from build123d import *

# Parameters (mm, degrees)
SKETCH1_W                = 50
SKETCH1_H                = 60
BOSS_EXTRUDE1_DEPTH      = 25
CUT_EXTRUDE1_START       = -16.25
SKETCH2_R                = 21
CUT_EXTRUDE1_DEPTH       = 17.5
CUT_EXTRUDE2_START       = -12
SKETCH3_R                = 7.5
CUT_EXTRUDE2_DEPTH       = 26
SKETCH4_R                = 5
CUT_EXTRUDE3_DEPTH       = 4
SKETCH10_W               = 11
SKETCH10_H               = 10
CUT_EXTRUDE9_DEPTH       = 11
SKETCH11_R               = 2.25
CUT_EXTRUDE10_DEPTH      = 50.398886627
SKETCH12_R               = 2
CUT_EXTRUDE11_DEPTH      = 50.371044145
SKETCH13_R               = 3.5
CUT_EXTRUDE12_DEPTH      = 50.371044145
CHAMFER1_SIZE            = 3
FILLET1_R                = 4
SKETCH14_R               = 1.8
CUT_EXTRUDE13_DEPTH      = 10
CUT_EXTRUDE14_DEPTH      = 7
BOSS_EXTRUDE2_DEPTH      = 5
CHAMFER2_SIZE            = 3
FILLET2_R                = 1
CUT_EXTRUDE15_DEPTH      = 66.030761952
CUT_EXTRUDE15_DEPTH_BACK = 66.030761952
SKETCH17_R               = 6
SKETCH21_R               = 7.75
CUT_EXTRUDE16_DEPTH      = 8
SKETCH22_W               = 20
SKETCH22_H               = 10
BOSS_EXTRUDE3_DEPTH      = 5
SKETCH23_R               = 3.25
CUT_EXTRUDE17_DEPTH      = 5
SKETCH24_R               = 5
CUT_EXTRUDE18_DEPTH      = 4
FILLET4_R                = 5
SKETCH25_R               = 1.5
CUT_EXTRUDE19_DEPTH      = 8
SKETCH26_R               = 3.6
CUT_EXTRUDE20_DEPTH      = 10


with BuildPart() as part:
    # Sketch1 → Boss-Extrude1 (new body)
    with BuildSketch(Plane(origin=(0, 0, 0), x_dir=(1, 0, 0), z_dir=(0, 1, 0))):
        Rectangle(SKETCH1_W, SKETCH1_H)
    extrude(amount=BOSS_EXTRUDE1_DEPTH)

    # Sketch2 → Cut-Extrude1 (cut)
    with BuildSketch(Plane.ZY.offset(25).offset(CUT_EXTRUDE1_START)):
        with Locations((0, 25)):
            Circle(SKETCH2_R)
    extrude(amount=-CUT_EXTRUDE1_DEPTH, mode=Mode.SUBTRACT)

    # Sketch3 → Cut-Extrude2 (cut)
    with BuildSketch(Plane.ZY.offset(25).offset(CUT_EXTRUDE2_START)):
        with Locations((0, 25)):
            Circle(SKETCH3_R)
    extrude(amount=-CUT_EXTRUDE2_DEPTH, mode=Mode.SUBTRACT)

    # Sketch4 → Cut-Extrude3 (cut)
    with BuildSketch(Plane.XY.offset(30)):
        with Locations((0, 25)):
            Circle(SKETCH4_R)
    extrude(amount=-CUT_EXTRUDE3_DEPTH, mode=Mode.SUBTRACT)

    # Sketch10 → Cut-Extrude9 (cut)
    with BuildSketch(Plane(origin=(25, 0, 0), x_dir=(0, 0, -1), z_dir=(1, 0, 0))):
        with Locations((-10, 5)):
            Rectangle(SKETCH10_W, SKETCH10_H)
        with Locations((10, 5)):
            Rectangle(SKETCH10_W, SKETCH10_H)
    cut_extrude9 = extrude(amount=-CUT_EXTRUDE9_DEPTH, mode=Mode.SUBTRACT)

    # Sketch11 → Cut-Extrude10 (cut, symmetric)
    with BuildSketch(Plane(origin=(0, 0, -4.5), x_dir=(-1, 0, 0), z_dir=(0, 0, -1))):
        with Locations(Location((-21, 5, 0), (0, 0, 90))):
            Circle(SKETCH11_R)
    cut_extrude10 = extrude(amount=CUT_EXTRUDE10_DEPTH, both=True, mode=Mode.SUBTRACT)

    # Mirror1: Cut-Extrude9, Cut-Extrude10 across plane
    add(cut_extrude9.mirror(Plane(origin=(0, 0, 0), x_dir=(0, 0, 1), z_dir=(1, 0, 0))), mode=Mode.SUBTRACT)
    add(cut_extrude10.mirror(Plane(origin=(0, 0, 0), x_dir=(0, 0, 1), z_dir=(1, 0, 0))), mode=Mode.SUBTRACT)

    # Sketch12 → Cut-Extrude11 (cut, symmetric)
    with BuildSketch(Plane(origin=(0, -2.5, 2.5), x_dir=(1, 0, 0), z_dir=(0, -0.7071067811865475, 0.7071067811865477))):
        with Locations(Location((20, 33.890872965, 0), (0, 0, 270))):
            Circle(SKETCH12_R)
        with Locations(Location((-20, 33.890872965, 0), (0, 0, 270))):
            Circle(SKETCH12_R)
    cut_extrude11 = extrude(amount=CUT_EXTRUDE11_DEPTH, both=True, mode=Mode.SUBTRACT)

    # Sketch13 → Cut-Extrude12 (cut, through all)
    with BuildSketch(Plane(origin=(0, -2.5, 2.5), x_dir=(1, 0, 0), z_dir=(0, -0.7071067811865475, 0.7071067811865477))):
        with Locations(Location((-20, 33.890872965, 0), (0, 0, 90))):
            Circle(SKETCH13_R)
        with Locations(Location((20, 33.890872965, 0), (0, 0, 90))):
            Circle(SKETCH13_R)
    cut_extrude12 = extrude(amount=CUT_EXTRUDE12_DEPTH, mode=Mode.SUBTRACT)

    # Mirror3: Cut-Extrude11, Cut-Extrude12 across plane
    add(cut_extrude11.mirror(Plane.XY), mode=Mode.SUBTRACT)
    add(cut_extrude12.mirror(Plane.XY), mode=Mode.SUBTRACT)

    # Chamfer1
    # the kernel refuses this chamfer: 3 mm, written as the material it takes off along each edge
    with BuildSketch(Plane(origin=(25, -7.715048964, -30), x_dir=(-1, 0, 0), z_dir=(0, 1, 0))) as chamfer1_piece_1:
        Polygon((CHAMFER1_SIZE, 0), (0, CHAMFER1_SIZE), (0, 0), align=None)
    extrude(amount=40.430097928, mode=Mode.SUBTRACT)
    with BuildSketch(Plane(origin=(-25, -7.715048964, -30), x_dir=(1, 0, 0), z_dir=(0, 1, 0))) as chamfer1_piece_2:
        Polygon((CHAMFER1_SIZE, 0), (0, -CHAMFER1_SIZE), (0, 0), align=None)
    extrude(amount=40.430097928, mode=Mode.SUBTRACT)

    # Fillet1
    fillet1_edges = [part.edges().sort_by_distance(p)[0] for p in [
        (-25, 10, -10),
        (25, 10, 10),
        (25, 10, -10),
        (-25, 10, 10),
    ]]
    fillet(fillet1_edges, radius=FILLET1_R)

    # Sketch14 → Cut-Extrude13 (cut)
    with BuildSketch(Plane.XZ):
        with Locations(Location((-15, -20.205680561, 0), (0, 0, 270))):
            Circle(SKETCH14_R)
        with Locations(Location((15, -20.205680561, 0), (0, 0, 270))):
            Circle(SKETCH14_R)
    extrude(amount=-CUT_EXTRUDE13_DEPTH, mode=Mode.SUBTRACT)

    # Sketch15 → Cut-Extrude14 (cut)
    with BuildSketch(Plane.XY.offset(30)):
        Polygon((-21, 0.958548116), (-17.5, 2.979274058), (-17.5, 7.020725942), (-21, 9.041451884), (-24.5, 7.020725942), (-24.5, 2.979274058), align=None)
        Polygon((21, 0.958548116), (24.5, 2.979274058), (24.5, 7.020725942), (21, 9.041451884), (17.5, 7.020725942), (17.5, 2.979274058), align=None)
    extrude(amount=-CUT_EXTRUDE14_DEPTH, mode=Mode.SUBTRACT)

    # Sketch16 → Boss-Extrude2 (add)
    with BuildSketch(Plane.XY.offset(30)):
        with BuildLine():
            Line((-25, 0), (-25, 9.464101615))
            Line((-25, 9.464101615), (-27, 6))
            Line((-27, 6), (-27, 1))
            ThreePointArc((-27, 1), (-26.707106781, 0.292893219), (-26, 0))
            Line((-26, 0), (-25, 0))
        make_face()
    boss_extrude2 = extrude(amount=-BOSS_EXTRUDE2_DEPTH)

    # Mirror4: Boss-Extrude2 across plane
    add(boss_extrude2.mirror(Plane(origin=(0, 0, 0), x_dir=(0, 0, 1), z_dir=(1, 0, 0))))

    # Chamfer2
    # the kernel refuses this chamfer: 3 mm, written as the material it takes off along each edge
    with BuildSketch(Plane(origin=(-25, 0, 25), x_dir=(0, 1, 0), z_dir=(0, 0, -1))) as chamfer2_piece_1:
        Polygon((CHAMFER2_SIZE, 0), (0, CHAMFER2_SIZE), (0, 0), align=None)
    extrude(amount=17.215048964, mode=Mode.SUBTRACT)
    with BuildSketch(Plane(origin=(-25, 0, 12.215048964), x_dir=(0, 1, 0), z_dir=(0, 0, -1))) as chamfer2_piece_2:
        Polygon((CHAMFER2_SIZE, 0), (0, CHAMFER2_SIZE), (0, 0), align=None)
    extrude(amount=24.430097928, mode=Mode.SUBTRACT)
    with BuildSketch(Plane(origin=(-25, 0, -7.784951036), x_dir=(0, 1, 0), z_dir=(0, 0, -1))) as chamfer2_piece_3:
        Polygon((CHAMFER2_SIZE, 0), (0, CHAMFER2_SIZE), (0, 0), align=None)
    extrude(amount=26.930097928, mode=Mode.SUBTRACT)
    with BuildSketch(Plane(origin=(-16.54463656, 0, -35.45536344), x_dir=(0, 1, 0), z_dir=(-0.7071067811865476, 0, 0.7071067811865476))) as chamfer2_piece_4:
        Polygon((CHAMFER2_SIZE, 0), (0, -CHAMFER2_SIZE), (0, 0), align=None)
    extrude(amount=19.672738615, mode=Mode.SUBTRACT)
    with BuildSketch(Plane(origin=(-29.715048964, 0, -30), x_dir=(0, 1, 0), z_dir=(1, 0, 0))) as chamfer2_piece_5:
        Polygon((CHAMFER2_SIZE, 0), (0, CHAMFER2_SIZE), (0, 0), align=None)
    extrude(amount=59.430097928, mode=Mode.SUBTRACT)
    with BuildSketch(Plane(origin=(16.54463656, 0, -35.45536344), x_dir=(0, 1, 0), z_dir=(0.7071067811865476, 0, 0.7071067811865476))) as chamfer2_piece_6:
        Polygon((CHAMFER2_SIZE, 0), (0, CHAMFER2_SIZE), (0, 0), align=None)
    extrude(amount=19.672738615, mode=Mode.SUBTRACT)
    with BuildSketch(Plane(origin=(25, 0, -34.715048964), x_dir=(-1, 0, 0), z_dir=(0, 0, 1))) as chamfer2_piece_7:
        Polygon((CHAMFER2_SIZE, 0), (0, -CHAMFER2_SIZE), (0, 0), align=None)
    extrude(amount=26.930097928, mode=Mode.SUBTRACT)
    with BuildSketch(Plane(origin=(25, 0, 7.784951036), x_dir=(-1, 0, 0), z_dir=(0, 0, 1))) as chamfer2_piece_8:
        Polygon((CHAMFER2_SIZE, 0), (0, -CHAMFER2_SIZE), (0, 0), align=None)
    extrude(amount=17.215048964, mode=Mode.SUBTRACT)
    with BuildSketch(Plane(origin=(25, 0, -12.215048964), x_dir=(-1, 0, 0), z_dir=(0, 0, 1))) as chamfer2_piece_9:
        Polygon((CHAMFER2_SIZE, 0), (0, -CHAMFER2_SIZE), (0, 0), align=None)
    extrude(amount=24.430097928, mode=Mode.SUBTRACT)

    # Fillet2
    fillet2_edges = [part.edges().sort_by_distance(p)[0] for p in [
        (-25, 6.232050808, 25),
        (25, 6.232050808, 25),
        (-23.5, 1.5, 25),
        (23.5, 1.5, 25),
    ]]
    fillet(fillet2_edges, radius=FILLET2_R)

    # Sketch17 → Cut-Extrude15 (cut, two sides: drawn at the far end of the back side and taken through both)
    with BuildSketch(Plane.ZY.offset(25).offset(-CUT_EXTRUDE15_DEPTH_BACK)):
        with Locations((0, 25)):
            Circle(SKETCH17_R)
    extrude(amount=CUT_EXTRUDE15_DEPTH + CUT_EXTRUDE15_DEPTH_BACK, mode=Mode.SUBTRACT)

    # Fillet3: read off the stored shape, not the designer's step
    # Fillet3 outline → Fillet3 (revolve, cut)
    with BuildSketch(Plane(origin=(0, 25, 0), x_dir=(0, 1, 0), z_dir=(0, 0, -1))):
        with BuildLine():
            Line((6, 25), (6, 17))
            ThreePointArc((6, 17), (8.343145751, 22.656854249), (14, 25))
            Line((14, 25), (6, 25))
        make_face()
        with BuildLine():
            ThreePointArc((14, -25), (8.343145751, -22.656854249), (6, -17))
            Line((6, -17), (6, -25))
            Line((6, -25), (14, -25))
        make_face()
    revolve(axis=Axis((0, 25, 0), (1, 0, 0)), mode=Mode.SUBTRACT)

    # Sketch21 → Cut-Extrude16 (cut)
    with BuildSketch(Plane.XY.offset(26)):
        with Locations((0, 25)):
            Circle(SKETCH21_R)
    extrude(amount=-CUT_EXTRUDE16_DEPTH, mode=Mode.SUBTRACT)

    # Sketch22 → Boss-Extrude3 (add)
    with BuildSketch(Plane.XY.offset(30)):
        with Locations((0, 20)):
            Rectangle(SKETCH22_W, SKETCH22_H)
    extrude(amount=BOSS_EXTRUDE3_DEPTH)

    # Sketch23 → Cut-Extrude17 (cut)
    with BuildSketch(Plane.XY.offset(35)):
        with Locations((0, 25)):
            Circle(SKETCH23_R)
    extrude(amount=-CUT_EXTRUDE17_DEPTH, mode=Mode.SUBTRACT)

    # Sketch24 → Cut-Extrude18 (cut)
    with BuildSketch(Plane.XY.offset(35)):
        with Locations((0, 25)):
            Circle(SKETCH24_R)
    extrude(amount=-CUT_EXTRUDE18_DEPTH, mode=Mode.SUBTRACT)

    # Fillet4
    fillet4_edges = [part.edges().sort_by_distance(p)[0] for p in [
        (-10, 20, 30),
        (0, 15, 30),
        (10, 20, 30),
    ]]
    fillet(fillet4_edges, radius=FILLET4_R - 0.0001)  # a hair under: the kernel refuses the full size

    # Sketch25 → Cut-Extrude19 (cut)
    with BuildSketch(Plane.XZ):
        with Locations(Location((10, 23, 0), (0, 0, 270))):
            Circle(SKETCH25_R)
        with Locations(Location((-10, 23, 0), (0, 0, 270))):
            Circle(SKETCH25_R)
        with Locations(Location((10, 13, 0), (0, 0, 270))):
            Circle(SKETCH25_R)
        with Locations(Location((-10, 13, 0), (0, 0, 270))):
            Circle(SKETCH25_R)
    extrude(amount=-CUT_EXTRUDE19_DEPTH, mode=Mode.SUBTRACT)

    # Sketch26 → Cut-Extrude20 (cut)
    with BuildSketch(Plane(origin=(0, 0, -30), x_dir=(-1, 0, 0), z_dir=(0, 0, -1))):
        with Locations((21, 5)):
            Circle(SKETCH26_R)
        with Locations((-21, 5)):
            Circle(SKETCH26_R)
    extrude(amount=-CUT_EXTRUDE20_DEPTH, mode=Mode.SUBTRACT)


solid = part.part
Design review of the part built by this model. Coordinates are the model's own, in mm. A direction names the side the tool comes from. Round coordinates to 2 decimals unless told otherwise and drop trailing zeros. One line per question, with ' | ' between items.
1. For L1, parallel to Z at x = -19, y = 3.5; L2, parallel to X at y = 5, z = -27; L3, parallel to X at y = 4.75, z = 13, list the stretches that pass through material, from the lowest coordinate up. Write a range as [from, to].
Results are:
L1: z = [-20, -15.5], [-4.5, 4.5], [15.5, 23] | L2: x = [-25, -24.6], [-17.4, 17.4], [24.6, 25] | L3: x = [-14, -11.5], [-8.5, 8.5], [11.5, 14]
2. We need section A-A, the plane z = 1.5. State how many separate pieces and enclosed holes the cut face has, and give its area (3 significant figures).
Results are:
separate pieces: 1 | enclosed holes: 2 | area: 613 mm²
3. Clearance check with flat-ended pins moving along their axes: P1, Ø11, axis at y = 3.5, z = -7.5, coming from the +X side; P2, Ø5.5, axis at x = -17, z = 11, coming from the -Y side; P3, Ø4, axis at x = -0.5, y = 22.5, coming from the +Z side. State where each tip first meets the part, or that it passes through.
Results are:
P1: stops at x = 25 | P2: stops at y = 10 | P3: stops at z = 31
4. Draft analysis for pull direction Y (two halves, no side actions). For faces 1 (the face through (18, 5, -15.5)), 2 (the face through (23.88, 1.46, 24.71)), 3 (the face through (19.2, 2, 26.5)), state which applies: released by +Y, released by -Y, zero draft, split by the parting line, or undercut.
Results are:
face 1: zero draft | face 2: released by -Y | face 3: undercut
5. For faces 4 (the face through (19.274, 8.045, 26.549)), 5 (the face through (-23, 7, -20)), 6 (the face through (18, 5, 4.5)), 7 (the face through (0, 7, 30)), list the 3-axis set-ups (+Z, -Z, +X, -X, +Y, -Y) from which the entire face can be reached by the end or side of a thin tool; tool diameter is ignored.
Results are:
face 4: +Z | face 5: -Z | face 6: +X, -Y | face 7: +Z, -Y
